Check sheet for the drawn part. Datum: minimum x, y, z corner. Units: mm. Coordinates: 2 decimals unless noted, no trailing zeros. Write each loop counter-clockwise with the first axis right and the second up, starting at its lowest first coordinate (ties: lowest second). Pieces come first, ordered by that corner, then holes. Notation, with made-up numbers: M 19.25,37 L 65.25,37 A24 cw 65.25,49 Z; hole C 88.5,28 d11. An arc over 180 degrees is marked long. Answer in a Markdown table with one row per item.
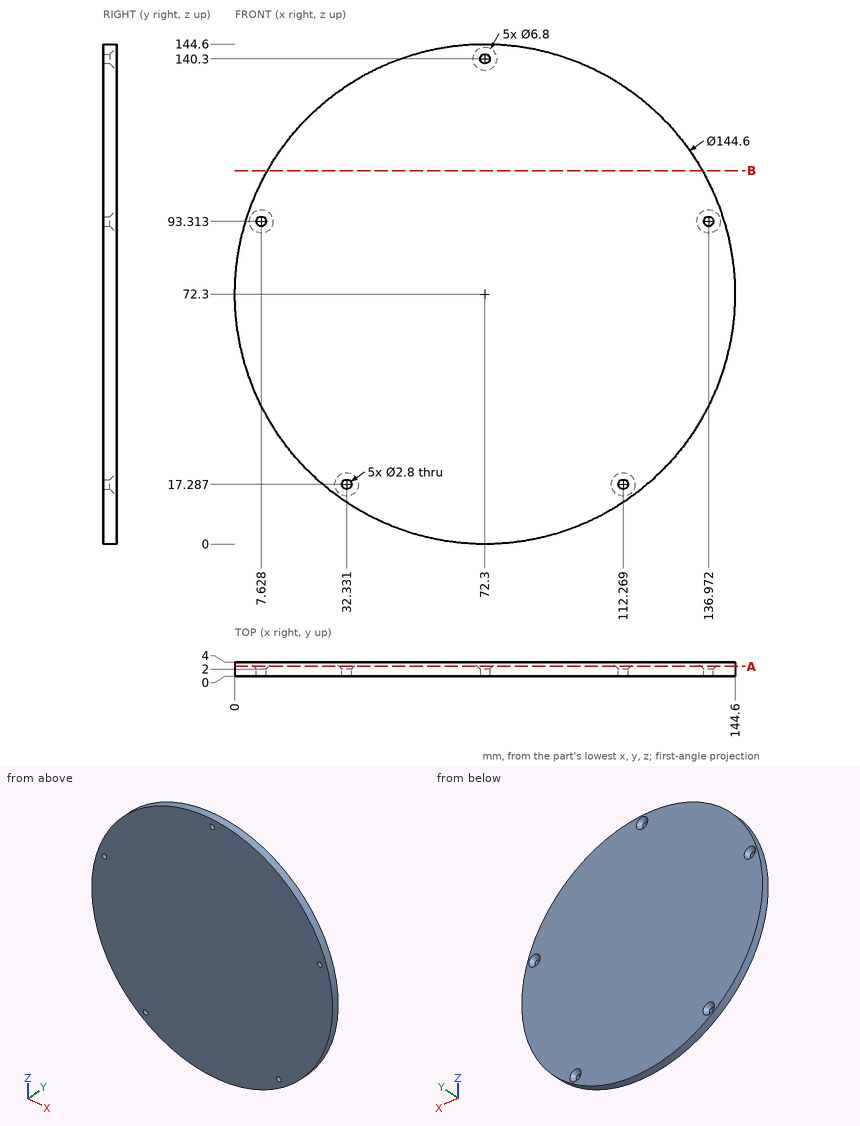
1) Sectioned sample at A-A (y = 2.8). Record the cut outline in (x, z).
Response values:
| item | result |
|---|---|
| outline | C 72.3,72.3 d144.6; hole C 7.63,93.31 d4.4; hole C 32.33,17.29 d4.4; hole C 72.3,140.3 d4.4; hole C 112.27,17.29 d4.4; hole C 136.97,93.31 d4.4 |
2) Depth check by flat-ended pin: pin 1 (4.5 mm diameter, centred on x = 72.3, z = 140.3, fed in from -Y); pin 2 (2 mm diameter, centred on x = 44.5, y = 0.5, fed in from -Z); pin 3 (1.5 mm diameter, centred on x = 70.5, y = 1.5, fed in from -Z); pin 4 (2.5 mm diameter, centred on x = 112.27, z = 17.29, fed in from -Y). Enter the tip coordinate at first touch or a pass-through.
Response values:
| item | result |
|---|---|
| pin 1 | stops at y = 0 |
| pin 2 | stops at z = 5.15 |
| pin 3 | stops at z = 0.01 |
| pin 4 | passes through |
3) Sectioned sample at B-B (z = 108). Record the cut outline in (x, y).
Response values:
| item | result |
|---|---|
| outline | M 9.43,0 L 135.17,0 L 135.17,4 L 9.43,4 Z |
4) Thickness scan on L1, parallel to Z at x = 112, y = 2.05 (1 decimal); L2, parallel to X at y = 0.75, z = 58; L3, parallel to X at y = 0.6, z = 128.5 (1 decimal). Record the ranges inside material, lowest first. Write a range as [from, to].
Response values:
| item | result |
|---|---|
| L1 | z = [11.9, 15.9], [18.7, 132.7] |
| L2 | x = [1.43, 143.17] |
| L3 | x = [26.8, 117.8] |
